from build123d import *

# Parameters (mm, degrees)
SKETCH1_W                   = 38.1
SKETCH1_H                   = 38.1
BOSS_EXTRUDE1_DEPTH         = 38.1
SKETCH4_R                   = 1.984375
CUT_EXTRUDE2_DEPTH          = 19.05
F_3_4_0_75_DIAMETER_HOLE1_D = 19.05


with BuildPart() as part:
    # Sketch1 → Boss-Extrude1 (new body)
    with BuildSketch(Plane.XY):
        with Locations((19.05, -19.05)):
            Rectangle(SKETCH1_W, SKETCH1_H)
    extrude(amount=BOSS_EXTRUDE1_DEPTH)

    # Sketch4 → Cut-Extrude2 (cut)
    with BuildSketch(Plane(origin=(0, 0, 0), x_dir=(1, 0, 0), z_dir=(0, 1, 0))):
        with Locations((6.35, -6.35)):
            Circle(SKETCH4_R)
        with Locations((6.35, -31.75)):
            Circle(SKETCH4_R)
        with Locations((31.75, -6.35)):
            Circle(SKETCH4_R)
        with Locations((31.75, -31.75)):
            Circle(SKETCH4_R)
    extrude(amount=-CUT_EXTRUDE2_DEPTH, mode=Mode.SUBTRACT)

    # 3/4 (0.75) Diameter Hole1 (through all)
    with Locations(Plane.XY.offset(38.1)):
        with Locations((19.05, -22.86)):
            Hole(F_3_4_0_75_DIAMETER_HOLE1_D / 2)


solid = part.part
Verification items for the finished model (mm, model axes). A direction names the side the tool comes from. Give positions to 0.01 mm unless a question says otherwise; leave off trailing zeros. Order: outer loops, then holes, each group sorted by start corner. A loop starts at its lowest first (then second) coordinate and runs counter-clockwise, first axis right, second up. Notation, with made-up numbers: M 23.5,-26.5 L 46.5,-26.5 A21 cw 46.5,-10.5 Z; hole C 32.25,76.5 d6. An arc over 180 degrees is marked long. Answer as a JSON object with one key per item and string values. Group by question number.
1) Cross-section at B-B (z = 6.35). Enter the section's corners in (x, y) (3 decimals).
2) Scan lines: line 1 along X through (y, z) = (-10.5, 6.35); line 2 along Z through (x, y) = (8, -19). Record each from-to range of solid material in increasing order. Write a range as [from, to].
3) Cross-section at C-C (x = 19.05). Enter the section's corners in (y, z) (3 decimals).
4) Mould release check, pull along Y, two halves, no side actions. Record for faces 1 (the face through (19, -38.1, 19)), 2 (the face through (38.1, -19, 19)), 3 (the face through (13.93, -14.83, 18.78)), 4 (the face through (19, 0, 19)): released by +Y, released by -Y, zero draft, split by the parting line, or undercut.
5) Cross-section at D-D (y = -14). Enter the section's corners in (x, z).
6) Access from +Z, -Z, +X, -X, +Y, -Y to the whole of each face (thin tool, end or side, straight path). Record for faces 5 (the face through (4.368, -9.392, 6.263)), 6 (the face through (19, -10, 0)).
7) Cross-section at A-A (y = -22.86). Enter the section's corners in (x, z) (3 decimals).
8) Depth check by flat-ended pin: pin 1 Ø2 at (x, z) = (6.5, 7) entering from +Y. Enter the tip coordinate at first touch or a pass-through.
Result sheet:
{
 "1": {"outline": "M 0,-38.1 L 38.1,-38.1 L 38.1,0 L 33.734,0 L 33.734,-19.05 L 29.766,-19.05 L 29.766,0 L 8.334,0 L 8.334,-19.05 L 4.366,-19.05 L 4.366,0 L 0,0 Z; hole C 19.05,-22.86 d19.05"},
 "2": {"line 1": "x = [0, 4.37], [8.33, 29.77], [33.73, 38.1]", "line 2": "z = [0, 5.25], [7.45, 30.65], [32.85, 38.1]"},
 "3": {"outline": "M -38.1,0 L -32.385,0 L -32.385,38.1 L -38.1,38.1 Z; M -13.335,0 L 0,0 L 0,38.1 L -13.335,38.1 Z"},
 "4": {"face 1": "released by -Y", "face 2": "zero draft", "face 3": "undercut", "face 4": "released by +Y"},
 "5": {"outline": "M 0,0 L 15.55,0 L 15.55,38.1 L 0,38.1 Z; M 22.55,0 L 38.1,0 L 38.1,38.1 L 22.55,38.1 Z; hole C 6.35,6.35 d3.97; hole C 6.35,31.75 d3.97; hole C 31.75,6.35 d3.97; hole C 31.75,31.75 d3.97"},
 "6": {"face 5": "+Y", "face 6": "-Z, +X, -X, +Y, -Y"},
 "7": {"outline": "M 0,0 L 9.525,0 L 9.525,38.1 L 0,38.1 Z; M 28.575,0 L 38.1,0 L 38.1,38.1 L 28.575,38.1 Z"},
 "8": {"pin 1": "stops at y = -19.05"}
}
